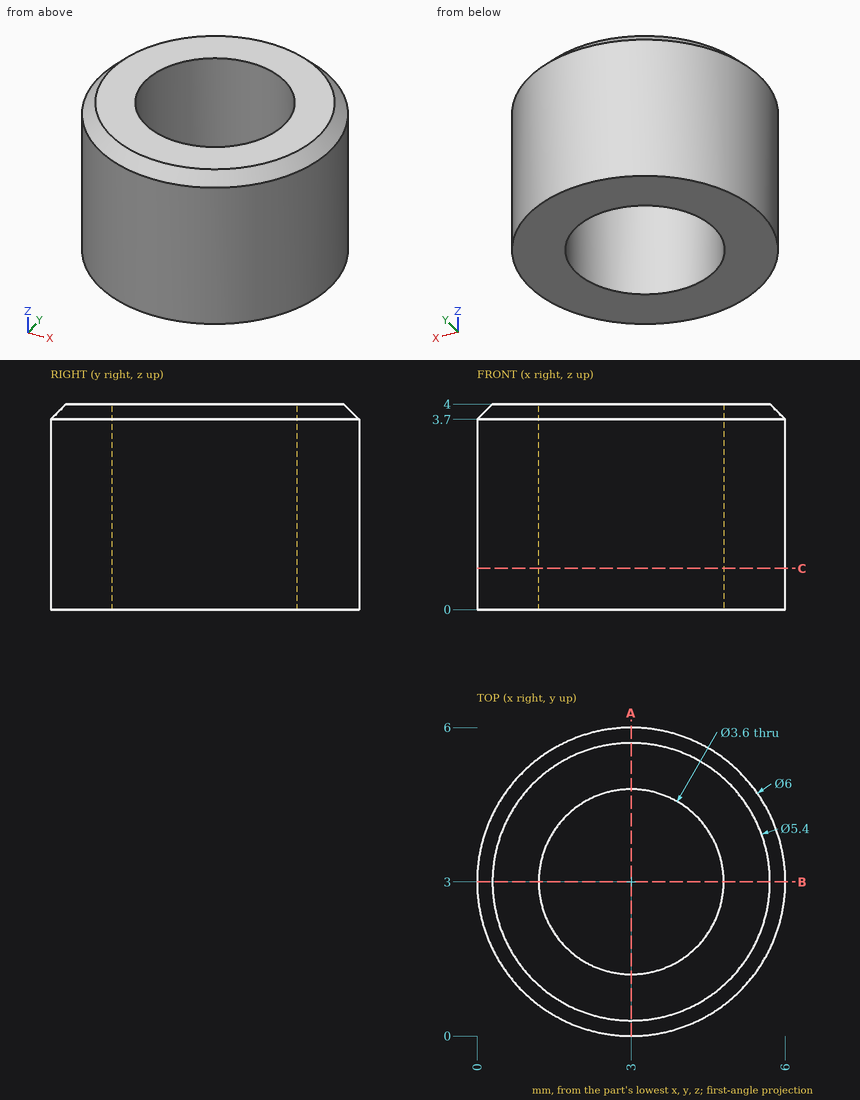
Drawing for the job (mm, zero at the part's lowest x, y, z). Round coordinates to 2 decimals unless told otherwise and drop trailing zeros. Loops run counter-clockwise (first coordinate to the right, second up) from the corner with the lowest first, then second, coordinate; pieces in that order, holes last.
1. Band-saw the part on C-C, the plane z = 0.8. List the corners of the cut face in (x, y).
Check values:
outline: circle Ø6 at (3, 3); hole circle Ø3.6 at (3, 3)
2. Drop flat-ended pins along their axis: P1, Ø1, axis at x = 1, z = 3, coming from the -Y side; P2, Ø1, axis at y = 1, z = 3, coming from the -X side. Give the stop position or say it passes through.
Check values:
P1: stops at y = 0.4
P2: stops at x = 0.4
3. Band-saw the part on A-A, the plane x = 3. List the corners of the cut face in (y, z), and give its area (3 significant figures).
Check values:
outline: (0, 0) - (1.2, 0) - (1.2, 4) - (0.3, 4) - (0, 3.7) - close; (4.8, 0) - (6, 0) - (6, 3.7) - (5.7, 4) - (4.8, 4) - close
area: 9.51 mm2
4. Wall check: probe 1 along Y at (x, z) = (3, 2.85); probe 2 along Y at (x, z) = (4, 1.7); probe 3 along X at (y, z) = (3.55, 3.2). Give the ranges that are in metal, low to high.
Check values:
probe 1: y = 0 to 1.2, 4.8 to 6
probe 2: y = 0.17 to 1.5, 4.5 to 5.83
probe 3: x = 0.05 to 1.29, 4.71 to 5.95
